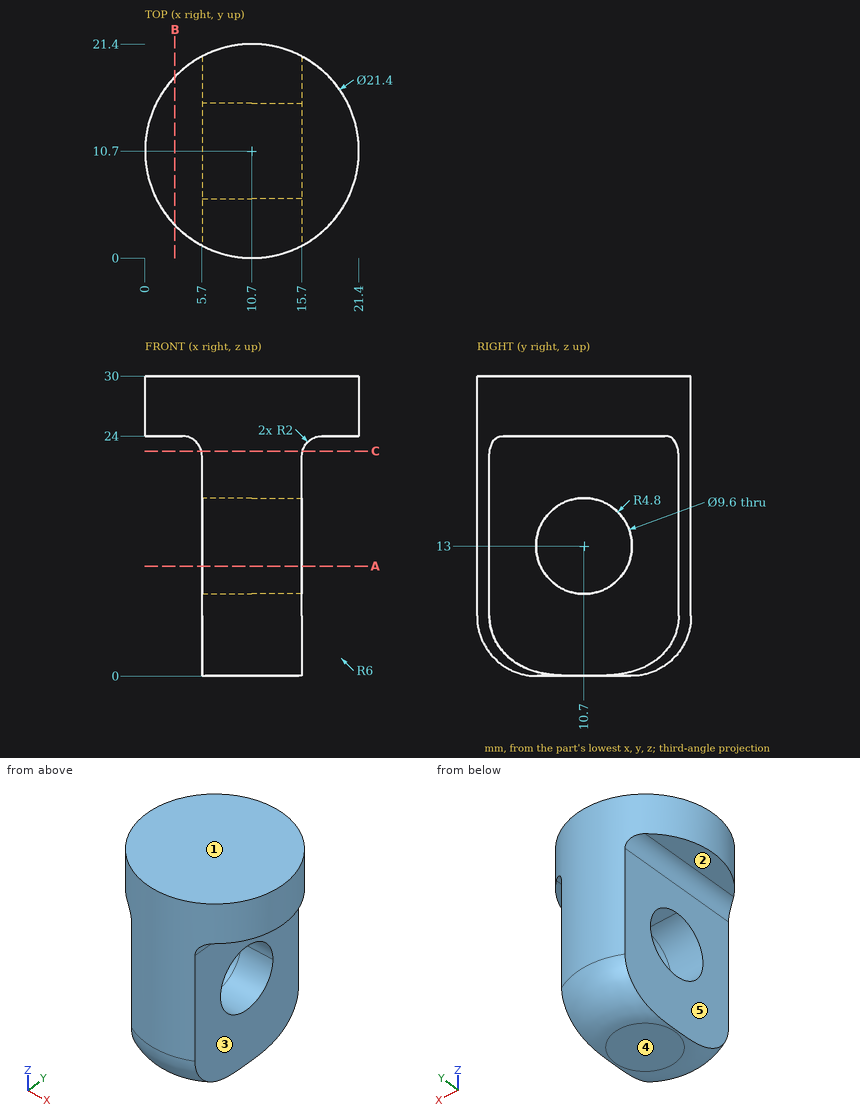
Could you check a few things on this drawing? It's one solid part, dimensions in mm from its lowest x, y, z. A direction names the side the tool comes from. Give positions to 0.01 mm unless a question says otherwise; leave off trailing zeros. Loops run counter-clockwise (first coordinate to the right, second up) from the corner with the lowest first, then second, coordinate; pieces in that order, holes last. Notation, with made-up numbers: (-35.5, -40) -> (7.5, -40) arc R26 ccw to (7.5, -18) -> close; hole circle Ø5 at (9, 84.25). An arc over 180 degrees is marked (long way). Answer as CSV lines item,"result". Start each with the question number.
(1) We'd pull the mould along Z, two halves only. Please class the marked faces 1, 2 and 3: released by +Z, released by -Z, zero draft, split by the parting line, or undercut.
(2) Which directions (+Z, -Z, +X, -X, +Y, -Y) give clear straight access to the entire face, cutting with the end or side of a thin tool? Please do the marked faces 4 and 5.
(3) I'm going to push flat-ended pins straight in: pin 1 Ø8 at (y, z) = (4.5, 22) entering from +X; pin 2 Ø6 at (x, y) = (15.5, 12) entering from -Z; pin 3 Ø4 at (y, z) = (6, 6.5) entering from -X; pin 4 Ø4 at (y, z) = (13.5, 23.5) entering from +X. Where does each tip first touch, or does it pass through?
(4) I need wall thicknesses on probe 1 along X at (y, z) = (13.5, 3); probe 2 along Y at (x, z) = (10.75, 14); probe 3 along Z at (x, y) = (11.75, 11). Which ranges of each line are inside material? Lowest first, please.
(5) If we section it at A-A on z = 11: Write out the boundary of the cut face in (x, y).
(6) If we section it at B-B on x = 3: Write out the boundary of the cut face in (y, z), then the cut area to 3 significant figures.
(7) If we section it at C-C on z = 22.5: Write out the boundary of the cut face in (x, y).
Computed:
1,face 1,"released by +Z"
1,face 2,"released by -Z"
1,face 3,"zero draft"
2,face 4,"-Z, +X, -X, +Y, -Y"
2,face 5,"-Z, -X, +Y, -Y"
3,pin 1,"stops at x = 21.04"
3,pin 2,"stops at z = 0"
3,pin 3,"stops at x = 5.7"
3,pin 4,"stops at x = 21.37"
4,probe 1,"x = 5.7 to 15.7"
4,probe 2,"y = 0 to 6.01, 15.39 to 21.4"
4,probe 3,"z = 0 to 8.21, 17.79 to 30"
5,outline,"(5.7, 1.24) arc R10.7 ccw to (15.7, 1.24) -> (15.7, 6.34) -> (5.7, 6.34) -> close; (5.7, 15.06) -> (15.7, 15.06) -> (15.7, 20.16) arc R10.7 ccw to (5.7, 20.16) -> close"
6,outline,"(3.27, 24) -> (18.13, 24) -> (18.13, 30) -> (3.27, 30) -> close"
6,area,"89.2 mm2"
7,outline,"(5.64, 1.27) arc R10.7 ccw to (15.76, 1.27) -> (15.76, 20.13) arc R10.7 ccw to (5.64, 20.13) -> close"
